from build123d import *

# Parameters (mm, degrees)
BOSS_EXTRUDE1_START = -1.5
SKETCH2_W           = 3.398401164
SKETCH2_H           = 2.43903778
BOSS_EXTRUDE1_DEPTH = 33.5
CIRPATTERN1_COUNT   = 12
CHAMFER1_SIZE       = 1


with BuildPart() as part:
    # Sketch1 → Revolve1 (revolve)
    with BuildSketch(Plane(origin=(0, 0, 0), x_dir=(1, 0, 0), z_dir=(0, 1, 0))):
        with BuildLine():
            Line((-44.863739249, 0), (76.664890153, 0))
            Line((76.664890153, 0), (76.664890153, 8.102912078))
            Line((76.664890153, 8.102912078), (74.664890153, 10.102912078))
            Line((74.664890153, 10.102912078), (18.02464627, 10.102912078))
            Line((18.02464627, 10.102912078), (16.52464627, 11.60370674))
            Line((16.52464627, 11.60370674), (5.800309153, 11.60370674))
            Line((5.800309153, 11.60370674), (4.300309153, 10.10370674))
            Line((4.300309153, 10.10370674), (4.300309153, 9.962333128))
            Line((4.300309153, 9.962333128), (-7.863739249, 9.962333128))
            ThreePointArc((-7.863739249, 9.962333128), (-9.277952812, 10.548119565), (-9.863739249, 11.962333128))
            Line((-9.863739249, 11.962333128), (-9.863739249, 12))
            Line((-9.863739249, 12), (-43.363739249, 12))
            Line((-43.363739249, 12), (-44.863739249, 10.5))
            Line((-44.863739249, 10.5), (-44.863739249, 0))
        make_face()
    revolve(axis=Axis((77.994791667, 0, 0), (-1, 0, 0)))

    # Sketch2 → Boss-Extrude1 (add)
    with BuildSketch(Plane.ZY.offset(44.921875).offset(BOSS_EXTRUDE1_START)):
        with Locations((0, 12.305085941)):
            Rectangle(SKETCH2_W, SKETCH2_H)
    boss_extrude1 = extrude(amount=-BOSS_EXTRUDE1_DEPTH)

    # CirPattern1: Boss-Extrude1 ×12 about axis
    cirpattern1_axis = Axis((0, 0, 0), (1, 0, 0))
    for i in range(1, CIRPATTERN1_COUNT):
        add(boss_extrude1.rotate(cirpattern1_axis, i * 360 / CIRPATTERN1_COUNT))

    # Chamfer1
    chamfer1_edges = [part.edges().sort_by_distance(p)[0] for p in [
        (-43.421875, -11.71265136, 6.762302416),
        (-43.421875, -13.524604831, 0),
        (-43.421875, -11.71265136, -6.762302416),
        (-43.421875, -6.762302416, -11.71265136),
        (-43.421875, 0, -13.524604831),
        (-43.421875, 6.762302416, -11.71265136),
        (-43.421875, 11.71265136, -6.762302416),
        (-43.421875, 13.524604831, 0),
        (-43.421875, 11.71265136, 6.762302416),
        (-43.421875, 6.762302416, 11.71265136),
        (-43.421875, 0, 13.524604831),
        (-43.421875, -6.762302416, 11.71265136),
    ]]
    chamfer(chamfer1_edges, length=CHAMFER1_SIZE)


solid = part.part
Work out the finished part from the listing and answer in its coordinate system (mm). A direction names the side the tool comes from. Round coordinates to 2 decimals unless told otherwise and drop trailing zeros. Loops run counter-clockwise (first coordinate to the right, second up) from the corner with the lowest first, then second, coordinate; pieces in that order, holes last. Notation, with made-up numbers: M 26.25,-28 L 37.25,-28 A35 cw 37.25,6 Z; hole C 62,80 d6. An arc over 180 degrees is marked long. One line per question, with ' | ' between items. Start each with the question number.
(1) Flat-ended cylindrical pins translate along their axes: pin 1 Ø1.5 at (x, y) = (38, -1.5) entering from -Z; pin 2 Ø2 at (x, y) = (-6, -9.5) entering from +Z; pin 3 Ø0.6 at (y, z) = (12, 0) entering from -X. Find the tip coordinate at first contact, or state that the pin passes through.
(2) Find the intervals of material crossed by line 1 (Y direction, x = 17, z = 7.5); line 2 (Z direction, x = -39, y = 6.25); line 3 (Y direction, x = 48.5, z = 6), in increasing order.
(3) A tool of negligible diameter and unlimited length cuts with its end or side. For faces 1 (the face through (-9.922, 11, -6)), 2 (the face through (-9.922, -6, 11)), 3 (the face through (-43.422, -6.1, 10.6)), from which of +Z, -Z, +X, -X, +Y, -Y can it reach the whole face along a straight path? Write none if from no direction.
(4) A cutting plane is placed at C-C on x = -5. Write down the section's boundary in (y, z), plus the area to 3 significant figures.
(5) A cutting plane is placed at D-D on x = 12. Write down the section's boundary in (y, z).
Geometry check:
1) pin 1: stops at z = -10.08 | pin 2: stops at z = 5.2 | pin 3: stops at x = -43.66
2) line 1: y = -8.22 to 8.22 | line 2: z = -12.01 to 12.01 | line 3: y = -8.13 to 8.13
3) face 1: -Z, +X, +Y | face 2: +Z, +X, -Y | face 3: +Z, -X, -Y
4) outline: C 0,0 d19.92 | area: 312 mm²
5) outline: C 0,0 d23.21
